from build123d import *

# Parameters (mm, degrees)
ESQUISSE1_R             = 5
BOSS_EXTRU_1_DEPTH      = 6
ESQUISSE2_R             = 3
BOSS_EXTRU_2_DEPTH      = 100
CHANFREIN1_SIZE         = 0.5
ENL_V_MAT_EXTRU_1_DEPTH = 3.5


with BuildPart() as part:
    # Esquisse1 → Boss.-Extru.1 (new body)
    with BuildSketch(Plane.XY):
        Circle(ESQUISSE1_R)
    extrude(amount=BOSS_EXTRU_1_DEPTH)

    # Esquisse2 → Boss.-Extru.2 (add)
    with BuildSketch(Plane.XY.offset(6)):
        Circle(ESQUISSE2_R)
    extrude(amount=BOSS_EXTRU_2_DEPTH)

    # Chanfrein1
    chanfrein1_edges = [part.edges().sort_by_distance(p)[0] for p in [
        (-3, 0, 106),
    ]]
    chamfer(chanfrein1_edges, length=CHANFREIN1_SIZE)

    # Esquisse3 → Enlèv. mat.-Extru.1 (cut)
    with BuildSketch(Plane(origin=(0, 0, 0), x_dir=(-1, 0, 0), z_dir=(0, 0, -1))):
        Polygon((-1.938814939, -2.138768329), (0.882820236, -2.748447155), (2.821635175, -0.609678826), (1.938814939, 2.138768329), (-0.882820236, 2.748447155), (-2.821635175, 0.609678826), align=None)
    extrude(amount=-ENL_V_MAT_EXTRU_1_DEPTH, mode=Mode.SUBTRACT)


solid = part.part
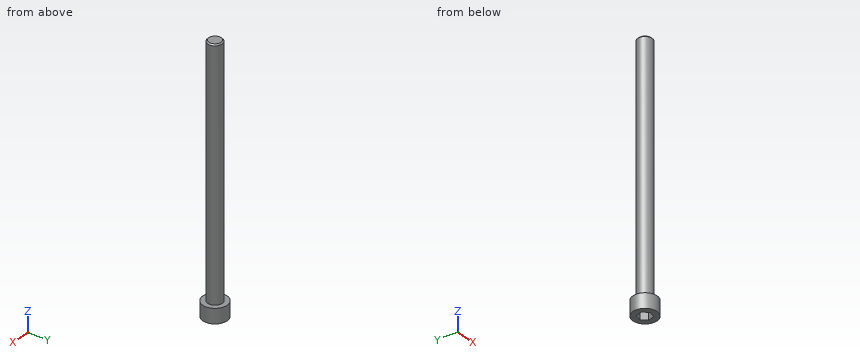
Model file for the job. Use its own axes, mm. Give positions to 0.01 mm unless a question says otherwise; leave off trailing zeros. Order: outer loops, then holes, each group sorted by start corner. A loop starts at its lowest first (then second) coordinate and runs counter-clockwise, first axis right, second up. Notation, with made-up numbers: M -1.5,-1 L 25.5,-1 A16 ccw 25.5,17 Z; hole C 29.25,78 d7. An arc over 180 degrees is marked long. Put each result on its own line as item: value. Start each with the question number.
(1) Pin check, flat tips, straight feed: pin 1 Ø6 at (y, z) = (-0.5, 63) entering from -X; pin 2 Ø1.5 at (x, y) = (-0.5, -2) entering from -Z; pin 3 Ø1.5 at (x, z) = (1.5, 45.5) entering from +Y; pin 4 Ø3 at (x, y) = (-3, 3.5) entering from +Z. Stop position of each tip, or through.
(2) Band-saw the part on A-A on z = 45. Give the cut face in (x, y).
(3) Drill centre lines: L1, parallel to Z at x = -4.5, y = -0.75; L2, parallel to Z at x = -0.5, y = 1; L3, parallel to X at y = -1.25, z = 28.5. Where is each one in solid material? Low to high. Write a range as [from, to].
(4) Band-saw the part on B-B on x = 0. Give the cut face in (y, z), then the cut area to 3 significant figures.
Results below:
1. pin 1: stops at x = -3
1. pin 2: stops at z = 0
1. pin 3: stops at y = 2.9
1. pin 4: stops at z = 6
2. outline: C 0,0 d6
3. L1: z = [0, 6]
3. L2: z = [3.5, 106]
3. L3: x = [-2.73, 2.73]
4. outline: M -5,0 L -2.56,0 L -2.56,3.5 L 2.56,3.5 L 2.56,0 L 5,0 L 5,6 L 3,6 L 3,105.5 L 2.5,106 L -2.5,106 L -3,105.5 L -3,6 L -5,6 Z
4. area: 642 mm2
